Read the model definition and answer for the solid it produces. Units are mm, in the model's axes. A direction names the side the tool comes from. Give positions to 0.01 mm unless a question says otherwise; leave off trailing zeros. Write each loop counter-clockwise with the first axis right and the second up, starting at its lowest first coordinate (ties: lowest second). Pieces come first, ordered by that corner, then holes.
Autodesk Inventor part; units mm, degrees
ref_plane "YZ Plane" through (0, 0, 0) normal (1, 0, 0) x (0, 1, 0)
ref_plane "XZ Plane" through (0, 0, 0) normal (0, 1, 0) x (-1, 0, 0)
ref_plane "XY Plane" through (0, 0, 0) normal (0, 0, 1) x (1, 0, 0)
sketch "Sketch1" plane through (0, 0, 0) normal (0, 0, 1) x (1, 0, 0)
  line L0 (-5, -6) -> (5, -6)
  line L1 (5, -6) -> (5, 6)
  line L2 (5, 6) -> (-5, 6)
  line L3 (-5, 6) -> (-5, -6)
  point P0 (0, 0)
  dimension "d0" = 10
  dimension "d1" = 12
  dimension "d2" = 5
  dimension "d3" = 6
extrude "Extrusion1" add sketch "Sketch1" along normal blind 25
sketch "Sketch2" plane through (0, 0, 25) normal (0, 0, 1) x (1, 0, 0)
  arc A0 (-1, -1.118) -> (-1, 1.118) centre (0, 0) ccw
  line L0 (-1, 1.118) -> (-1, -1.118)
  dimension "d6" = 3
extrude "Extrusion2" add sketch "Sketch2" along normal blind 9.27
properties part number "Motor"
Item 1: Which of the six approach directions +Z, -Z, +X, -X, +Y, -Y give full straight-line access (tool end or side, diameter ignored) to faces 1 (the flat face through (-5, 0, 12)), 2 (the flat face through (-1, 0, 30)), 3 (the cylindrical face through (1.5, 0, 29.6))?
Result set:
face 1: +Z, -Z, -X, +Y, -Y
face 2: +Z, -X, +Y, -Y
face 3: +Z
Item 2: Section A-A (x = 1) is taken. Write down the section's boundary in (y, z), and give its area (3 significant figures).
Result set:
outline: (-6, 0) - (6, 0) - (6, 25) - (1.12, 25) - (1.12, 34.27) - (-1.12, 34.27) - (-1.12, 25) - (-6, 25) - close
area: 321 mm2
Item 3: Find the intervals of material crossed by line 1 along Z through (x, y) = (-1, -1.25), in increasing order.
Result set:
line 1: z = 0 to 25
Item 4: Determine the mould class of faces 4 (the flat face through (0, -6, 12)), 5 (the flat face through (0, 0, 34.27)), 6 (the flat face through (0, 6, 12)) for opening direction Y: pulls with the +Y half, pulls with the -Y half, needs draft (parallel to the pull), parting line crosses it, or undercut.
Result set:
face 4: pulls with the -Y half
face 5: needs draft
face 6: pulls with the +Y half
Item 5: Section C-C (z = 29) is taken. Write down the section's boundary in (x, y), and give its area (3 significant figures).
Result set:
outline: (-1, -1.12) arc R1.5 ccw (long way) to (-1, 1.12) - close
area: 6.29 mm2
Item 6: This flat-tipped pin is pushed along its axis until it touches: pin 1 Ø1.8 at (y, z) = (0, 28) entering from -X. Where does it stop, or does it pass through?
Result set:
pin 1: stops at x = -1
Item 7: Section B-B (y = 0) is taken. Write down the section's boundary in (x, z).
Result set:
outline: (-5, 0) - (5, 0) - (5, 25) - (1.5, 25) - (1.5, 34.27) - (-1, 34.27) - (-1, 25) - (-5, 25) - close
Item 8: Section D-D (x = -1.5) is taken. Write down the section's boundary in (y, z).
Result set:
outline: (-6, 0) - (6, 0) - (6, 25) - (-6, 25) - close
